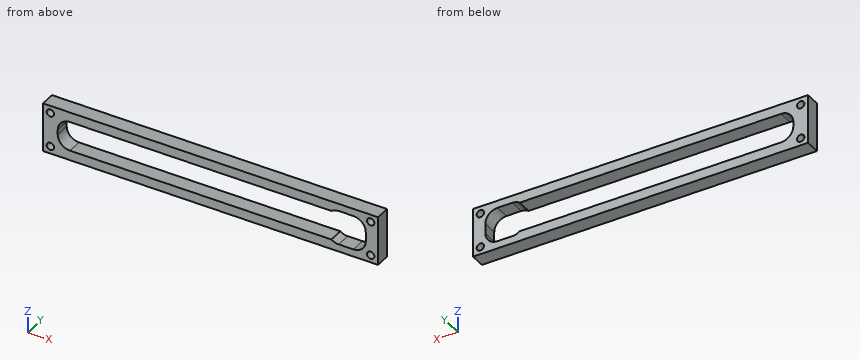
```python
from build123d import *

# Parameters (mm, degrees)
SKETCH1_W           = 136.427821805
SKETCH1_H           = 20
SKETCH1_R           = 1.5
SKETCH1_W_2         = 124.427821805
SKETCH1_H_2         = 12
BOSS_EXTRUDE1_DEPTH = 6
CUT_EXTRUDE1_DEPTH  = 139.01648656
FILLET1_R           = 5


with BuildPart() as part:
    # Sketch1 → Boss-Extrude1 (new body)
    with BuildSketch(Plane(origin=(0, 0, 0), x_dir=(1, 0, 0), z_dir=(0, 1, 0))):
        with Locations((68.213910903, 10)):
            Rectangle(SKETCH1_W, SKETCH1_H)
        with Locations(Location((3, 17, 0), (0, 0, 270))):
            Circle(SKETCH1_R, mode=Mode.SUBTRACT)
        with Locations(Location((3, 3, 0), (0, 0, 90))):
            Circle(SKETCH1_R, mode=Mode.SUBTRACT)
        with Locations(Location((133.427821805, 3, 0), (0, 0, 270))):
            Circle(SKETCH1_R, mode=Mode.SUBTRACT)
        with Locations(Location((133.427821805, 17, 0), (0, 0, 90))):
            Circle(SKETCH1_R, mode=Mode.SUBTRACT)
        with Locations((68.213910903, 10)):
            Rectangle(SKETCH1_W_2, SKETCH1_H_2, mode=Mode.SUBTRACT)
    extrude(amount=BOSS_EXTRUDE1_DEPTH)

    # Sketch2 → Cut-Extrude1 (cut, through all)
    with BuildSketch(Plane(origin=(0, 6, 0), x_dir=(1, 0, 0), z_dir=(0, 1, 0))):
        Polygon((117.427821805, 17), (117.427821805, 16), (130.427821805, 16), (130.427821805, 4), (117.427821805, 4), (117.427821805, 3), (131.427821805, 3), (131.427821805, 17), align=None)
    extrude(amount=-CUT_EXTRUDE1_DEPTH, mode=Mode.SUBTRACT)

    # Fillet1
    # the kernel refuses this fillet: 5 mm, written as the material it adds along each edge
    with BuildSketch(Plane(origin=(131.427821805, 6, -17), x_dir=(0, 0, 1), z_dir=(0, -1, 0)), Plane(origin=(131.427821805, 6, -3), x_dir=(-1, 0, 0), z_dir=(0, -1, 0)), Plane(origin=(6, 0, -16), x_dir=(0, 0, 1), z_dir=(0, 1, 0))) as fillet1_piece_1:
        with BuildLine():
            CenterArc((FILLET1_R, FILLET1_R), FILLET1_R, 180, 90)
            Line((0, FILLET1_R), (-FILLET1_R * 0.02, FILLET1_R))
            Line((-FILLET1_R * 0.02, FILLET1_R), (-FILLET1_R * 0.02, -FILLET1_R * 0.02))
            Line((-FILLET1_R * 0.02, -FILLET1_R * 0.02), (FILLET1_R, -FILLET1_R * 0.02))
            Line((FILLET1_R, -FILLET1_R * 0.02), (FILLET1_R, 0))
        make_face()
    extrude(amount=6)
    with BuildSketch(Plane(origin=(117.427821805, 6, -17), x_dir=(1, 0, 0), z_dir=(0, -1, 0))) as fillet1_piece_2:
        with BuildLine():
            CenterArc((3, 5), FILLET1_R, 233.130102354, 36.869897646)
            Line((0, 1), (-0.06, 0.92))
            ThreePointArc((-0.06, 0.92), (-0.1, 0.5), (-0.1, 0))
            Line((-0.1, 0), (0, -0.1))
            Line((0, -0.1), (3, -0.1))
            Line((3, -0.1), (3, 0))
        make_face()
    extrude(amount=6)
    with BuildSketch(Plane(origin=(117.427821805, 6, -3), x_dir=(0, 0, -1), z_dir=(0, -1, 0))) as fillet1_piece_3:
        with BuildLine():
            CenterArc((5, 3), FILLET1_R, 180, 36.869897646)
            Line((0, 3), (-0.1, 3))
            Line((-0.1, 3), (-0.1, 0))
            Line((-0.1, 0), (0, -0.1))
            ThreePointArc((0, -0.1), (0.5, -0.1), (0.92, -0.06))
            Line((0.92, -0.06), (1, 0))
        make_face()
    extrude(amount=6)
    with BuildSketch(Plane(origin=(6, 0, -4), x_dir=(0, 0, -1), z_dir=(0, 1, 0))) as fillet1_piece_4:
        with BuildLine():
            CenterArc((FILLET1_R, -FILLET1_R), FILLET1_R, 90, 90)
            Line((0, -FILLET1_R), (-FILLET1_R * 0.02, -FILLET1_R))
            Line((-FILLET1_R * 0.02, -FILLET1_R), (-FILLET1_R * 0.02, FILLET1_R * 0.02))
            Line((-FILLET1_R * 0.02, FILLET1_R * 0.02), (FILLET1_R, FILLET1_R * 0.02))
            Line((FILLET1_R, FILLET1_R * 0.02), (FILLET1_R, 0))
        make_face()
    extrude(amount=6)


solid = part.part
```
For this review, take the finished solid that the model builds, in its own axes (mm). Coordinates: 2 decimals unless noted, no trailing zeros. Order: outer loops, then holes, each group sorted by start corner. A loop starts at its lowest first (then second) coordinate and runs counter-clockwise, first axis right, second up. Notation, with made-up numbers: (60.5, 5.25) -> (102.5, 5.25) arc R34 cw to (102.5, 44.25) -> close; hole circle Ø6 at (3.5, 59). An arc over 180 degrees is marked (long way). Answer as CSV lines item,"result".
Q1. We need section D-D (y = 1.3). State the section outline as (x, z) points, plus the area to 3 significant figures.
Model answer:
outline,"(0, -20) -> (136.43, -20) -> (136.43, 0) -> (0, 0) -> close; hole circle Ø3 at (3, -17); hole circle Ø3 at (3, -3); hole (6, -11) arc R5 ccw to (11, -16) -> (117.43, -16) arc R5 ccw to (120.43, -17) -> (126.43, -17) arc R5 ccw to (131.43, -12) -> (131.43, -8) arc R5 ccw to (126.43, -3) -> (120.43, -3) arc R5 ccw to (117.43, -4) -> (11, -4) arc R5 ccw to (6, -9) -> close; hole circle Ø3 at (133.43, -17); hole circle Ø3 at (133.43, -3)"
area,"1,190 mm2"
Q2. We need section A-A (x = 3). State the section outline as (y, z) points.
Model answer:
outline,"(0, -20) -> (6, -20) -> (6, -18.5) -> (0, -18.5) -> close; (0, -15.5) -> (6, -15.5) -> (6, -4.5) -> (0, -4.5) -> close; (0, -1.5) -> (6, -1.5) -> (6, 0) -> (0, 0) -> close"
Q3. We need section C-C (x = 69). State the section outline as (y, z) points, plus the area to 3 significant figures.
Model answer:
outline,"(0, -20) -> (6, -20) -> (6, -16) -> (0, -16) -> close; (0, -4) -> (6, -4) -> (6, 0) -> (0, 0) -> close"
area,"48.0 mm2"
Q4. Clearance check with flat-ended pins moving along their axes: pin 1 Ø3.5 at (x, z) = (133.43, -3) entering from -Y; pin 2 Ø2.5 at (x, z) = (3, -3) entering from +Y. State where each tip first meets the part, or that it passes through.
Model answer:
pin 1,"stops at y = 0"
pin 2,"passes through"
Q5. We need section B-B (z = -14.25). State the section outline as (x, y) points.
Model answer:
outline,"(0, 0) -> (7.2, 0) -> (7.2, 6) -> (0, 6) -> close; (130.89, 0) -> (136.43, 0) -> (136.43, 6) -> (130.89, 6) -> close"
Q6. Wall thickness on line 1 along Z through (x, y) = (52.5, 4.3); line 2 along Z through (x, y) = (119.5, 5.2); line 3 along X through (y, z) = (5.15, -8.25): over which ranges is each line inside the solid? List them lowest first. Write a range as [from, to].
Model answer:
line 1,"z = [-20, -16], [-4, 0]"
line 2,"z = [-20, -16.91], [-3.09, 0]"
line 3,"x = [0, 6.06], [131.43, 136.43]"
